Check sheet for the modelled part. Datum: model origin and axes. Units: mm. Round coordinates to 2 decimals unless told otherwise and drop trailing zeros. Order: outer loops, then holes, each group sorted by start corner. A loop starts at its lowest first (then second) coordinate and runs counter-clockwise, first axis right, second up. Notation, with made-up numbers: M 9.5,24 L 45.5,24 A16 ccw 45.5,53 Z; hole C -17,-0.75 d8. An arc over 180 degrees is marked long. One line per item, written item: value. Start each with the question number.
(1) Depth check by flat-ended pin: pin 1 Ø2 at (y, z) = (-57, 1.5) entering from +X; pin 2 Ø1.5 at (y, z) = (54.5, 6.5) entering from -X; pin 3 Ø8 at (x, y) = (45, 0) entering from +Z; pin 4 Ø1 at (x, z) = (31.5, 3.5) entering from +Y. Enter the tip coordinate at first touch or a pass-through.
(2) Cross-section at B-B, the plane x = -45. Enter the section's corners in (y, z), and give its area (3 significant figures).
(3) Thickness scan on L1, parallel to Y at x = -27.5, z = 4.75; L2, parallel to Y at x = 20, z = 4.5; L3, parallel to Y at x = 49, z = 4. Record the ranges inside material, lowest first.
(4) Cross-section at C-C, the plane z = 3.25. Count the separate pieces of the cut face and the enclosed holes in it, and give its area (3 significant figures).
(5) Release check for a two-part mould opening along X. For faces 1 (the face through (24.864, 1.532, 4.056)), 2 (the face through (-1, 1, 8)), 3 (the face through (-67.453, -51.721, 3.944)) record: released by +X, released by -X, zero draft, split by the parting line, or undercut.
(6) Cross-section at A-A, the plane y = 0. Enter the section's corners in (x, z), and give its area (3 significant figures).
from build123d import *

# Parameters (mm, degrees)
SKETCH_1_R          = 85
SKETCH_1_R_2        = 3
EXTRUDE_1_DEPTH     = 8
SKETCH_2_R          = 5.1
CUT_EXTRUDE_1_DEPTH = 121.474063599


with BuildPart() as part:
    # 草图1 → 凸台-拉伸1 (new body)
    with BuildSketch(Plane.XY):
        Circle(SKETCH_1_R)
        with Locations((0, 75)):
            Circle(SKETCH_1_R_2, mode=Mode.SUBTRACT)
        with Locations((64.951905284, 37.5)):
            Circle(SKETCH_1_R_2, mode=Mode.SUBTRACT)
        with Locations((64.951905284, -37.5)):
            Circle(SKETCH_1_R_2, mode=Mode.SUBTRACT)
        with Locations((0, -75)):
            Circle(SKETCH_1_R_2, mode=Mode.SUBTRACT)
        with Locations((-64.951905284, -37.5)):
            Circle(SKETCH_1_R_2, mode=Mode.SUBTRACT)
        with Locations((-64.951905284, 37.5)):
            Circle(SKETCH_1_R_2, mode=Mode.SUBTRACT)
    extrude(amount=EXTRUDE_1_DEPTH)

    # 草图2 → 切除-拉伸1 (cut, through all)
    with BuildSketch(Plane.XY.offset(8)):
        with Locations((0, 45)):
            Circle(SKETCH_2_R)
        with Locations((31.819805153, 31.819805153)):
            Circle(SKETCH_2_R)
        with Locations((45, 0)):
            Circle(SKETCH_2_R)
        with Locations((31.819805153, -31.819805153)):
            Circle(SKETCH_2_R)
        with Locations((0, -45)):
            Circle(SKETCH_2_R)
        with Locations((-31.819805153, -31.819805153)):
            Circle(SKETCH_2_R)
        with Locations((-45, 0)):
            Circle(SKETCH_2_R)
        with Locations((-31.819805153, 31.819805153)):
            Circle(SKETCH_2_R)
        with Locations((0, 20)):
            Circle(SKETCH_2_R)
        with Locations((20, 0)):
            Circle(SKETCH_2_R)
        with Locations((0, -20)):
            Circle(SKETCH_2_R)
        with Locations((-20, 0)):
            Circle(SKETCH_2_R)
    extrude(amount=-CUT_EXTRUDE_1_DEPTH, mode=Mode.SUBTRACT)


solid = part.part
Values found:
1. pin 1: x = 63.95
1. pin 2: x = -65.85
1. pin 3: through
1. pin 4: y = 79.15
2. outline: M -72.11,0 L -5.1,0 L -5.1,8 L -72.11,8 Z; M 5.1,0 L 72.11,0 L 72.11,8 L 5.1,8 Z
2. area: 1,070 mm^2
3. L1: -80.43 to -34.53, -29.11 to 29.11, 34.53 to 80.43
3. L2: -82.61 to -5.1, 5.1 to 82.61
3. L3: -69.46 to -3.16, 3.16 to 69.46
4. separate pieces: 1
4. enclosed holes: 18
4. area: 21,500 mm^2
5. face 1: undercut
5. face 2: zero draft
5. face 3: split by the parting line
6. outline: M -85,0 L -50.1,0 L -50.1,8 L -85,8 Z; M -39.9,0 L -25.1,0 L -25.1,8 L -39.9,8 Z; M -14.9,0 L 14.9,0 L 14.9,8 L -14.9,8 Z; M 25.1,0 L 39.9,0 L 39.9,8 L 25.1,8 Z; M 50.1,0 L 85,0 L 85,8 L 50.1,8 Z
6. area: 1,030 mm^2
